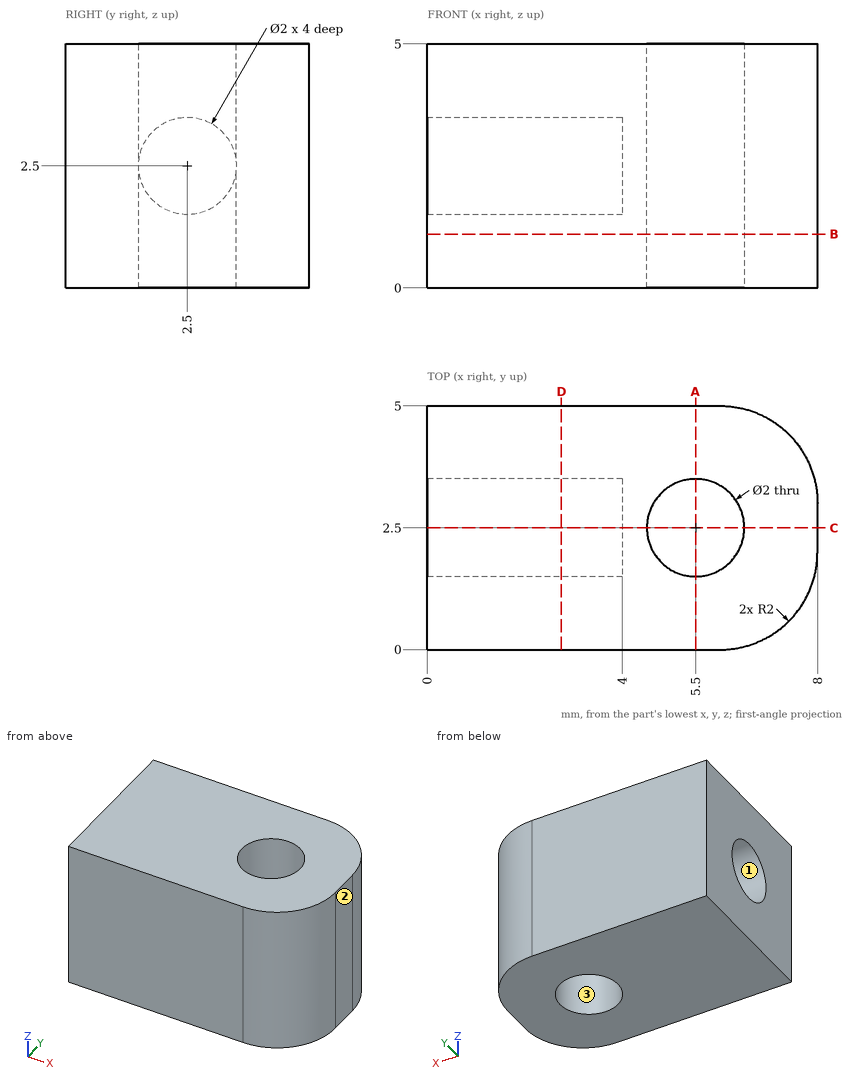
Job drawing, mm, ordinate dimensions from the low corner. One solid piece. Coordinates: 2 decimals unless noted, no trailing zeros. Write each loop counter-clockwise with the first axis right and the second up, starting at its lowest first coordinate (ties: lowest second). Pieces come first, ordered by that corner, then holes. Notation, with made-up numbers: M 19,7 L 41,7 A18 cw 41,35 Z; hole C 47,83.25 d11. An arc over 180 degrees is marked long. Answer as a JSON object with one key per item and string values. Group by question number.
1) Saw through at B-B (z = 1.1). Write the cut outline in (x, y), plus the area to 3 significant figures.
2) Saw through at A-A (x = 5.5). Write the cut outline in (y, z), plus the area to 3 significant figures.
3) Saw through at C-C (y = 2.5). Write the cut outline in (x, z), plus the area to 3 significant figures.
4) Pin check, flat tip, straight feed: pin 1 Ø1.8 at (x, y) = (5.5, 2.5) entering from -Z. Stop position of the tip, or through.
5) Saw through at D-D (x = 2.75). Write the cut outline in (y, z).
6) Wall check: line 1 (Y direction, x = 2.3, z = 2.5); line 2 (Z direction, x = 3.5, y = 2.85); line 3 (X direction, y = 2.75, z = 0.9). Give the ranges that are in metal, low to high. Write a range as from..to.
7) Mould opens along X. For the marked faces 1, 2 and 3 say: +X half, -X half, draft (parallel to the pull), parting line (faces both ways), or undercut.
Values follow:
{
 "1": {"outline": "M 0,0 L 6,0 A2 ccw 8,2 L 8,3 A2 ccw 6,5 L 0,5 Z; hole C 5.5,2.5 d2", "area": "35.1 mm2"},
 "2": {"outline": "M 0,0 L 1.5,0 L 1.5,5 L 0,5 Z; M 3.5,0 L 5,0 L 5,5 L 3.5,5 Z", "area": "15.0 mm2"},
 "3": {"outline": "M 0,0 L 4.5,0 L 4.5,5 L 0,5 L 0,3.5 L 4,3.5 L 4,1.5 L 0,1.5 Z; M 6.5,0 L 8,0 L 8,5 L 6.5,5 Z", "area": "22.0 mm2"},
 "4": {"pin 1": "passes through"},
 "5": {"outline": "M 0,0 L 5,0 L 5,5 L 0,5 Z; hole C 2.5,2.5 d2"},
 "6": {"line 1": "y = 0..1.5, 3.5..5", "line 2": "z = 0..1.56, 3.44..5", "line 3": "x = 0..4.53, 6.47..8"},
 "7": {"face 1": "draft", "face 2": "+X half", "face 3": "undercut"}
}
